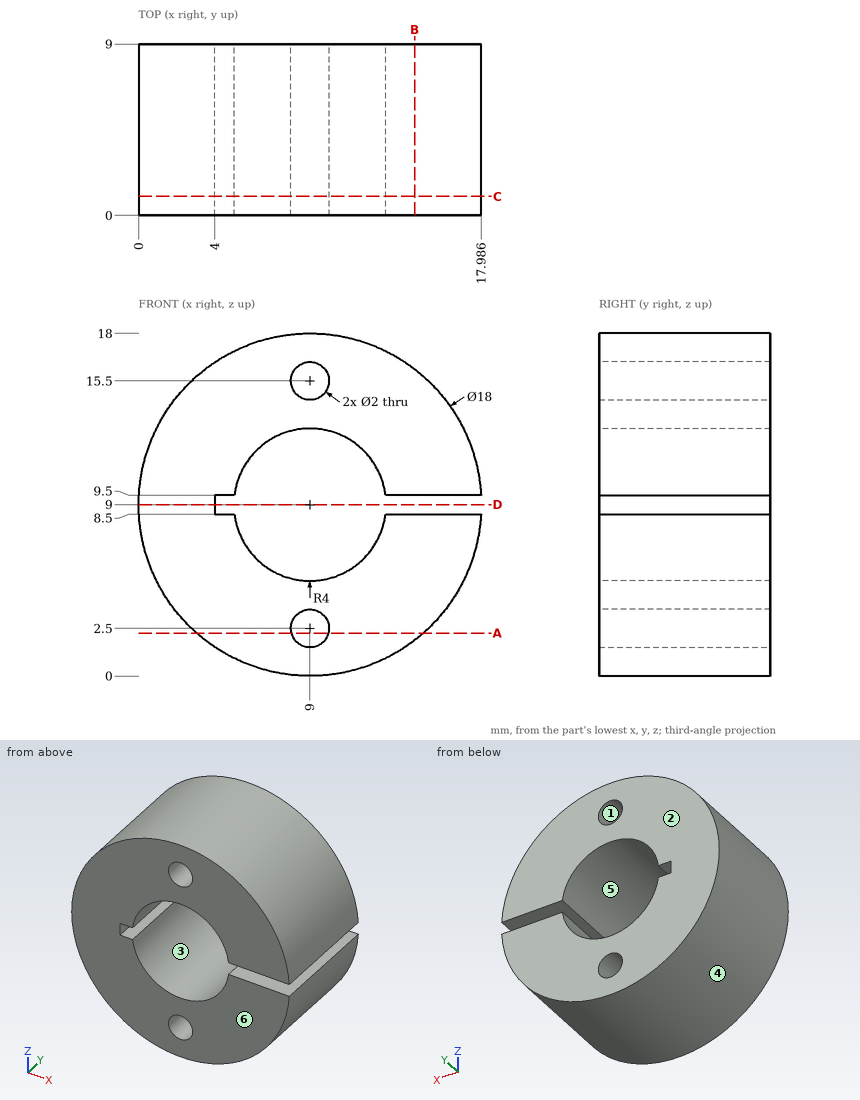
Verification items for this drawing (mm, ordinates from the low corner). A direction names the side the tool comes from. Coordinates: 2 decimals unless noted, no trailing zeros. Loops run counter-clockwise (first coordinate to the right, second up) from the corner with the lowest first, then second, coordinate; pieces in that order, holes last.
Item 1: Access from +Z, -Z, +X, -X, +Y, -Y to the whole of each face (thin tool, end or side, straight path). Record for the marked faces 5 and 6.
Item 2: Sectioned sample at B-B, the plane x = 14.5. Record the boundary of the cut face in (y, z), then the cut area to 3 significant figures.
Item 3: Release check for a two-part mould opening along X. For the marked faces 1, 2, 3 and 4 record: released by +X, released by -X, zero draft, split by the parting line, or undercut.
Item 4: Sectioned sample at D-D, the plane z = 9. Record the boundary of the cut face in (x, y).
Item 5: Sectioned sample at C-C, the plane y = 1. Record the boundary of the cut face in (x, z).
Item 6: Sectioned sample at A-A, the plane z = 2.25. Record the boundary of the cut face in (x, y), then the cut area to 3 significant figures.
Item 7: Go/stop test with flat-tipped pins: pin 1 Ø5 at (y, z) = (1.5, 14.5) entering from +X; pin 2 Ø2.5 at (x, z) = (9, 15.5) entering from -Y; pin 3 Ø1.5 at (x, y) = (15, 6.5) entering from +Z; pin 4 Ø0.8 at (y, z) = (5.5, 9) entering from +X. Record where each tip stops, or that it passes through.
Item 8: Thickness scan on line 1 (Z direction, x = 8.25, y = 5.75); line 2 (Z direction, x = 8.5, y = 3.5); line 3 (X direction, y = 2.5, z = 15.5) (1 decimal). Record the ranges inside material, lowest first.
Check result:
1. face 5: +Y, -Y
1. face 6: +Z, -Z, +X, -X, -Y
2. outline: (0, 1.88) - (9, 1.88) - (9, 8.5) - (0, 8.5) - close; (0, 9.5) - (9, 9.5) - (9, 16.12) - (0, 16.12) - close
2. area: 119 mm2
3. face 1: undercut
3. face 2: zero draft
3. face 3: undercut
3. face 4: split by the parting line
4. outline: (0, 0) - (4, 0) - (4, 9) - (0, 9) - close
5. outline: (4, 8.5) - (4, 9.5) - (5.03, 9.5) arc R4 cw to (12.97, 9.5) - (17.99, 9.5) arc R9 ccw (long way) to (17.99, 8.5) - (12.97, 8.5) arc R4 cw to (5.03, 8.5) - close; hole circle Ø2 at (9, 2.5); hole circle Ø2 at (9, 15.5)
6. outline: (3.05, 0) - (8.03, 0) - (8.03, 9) - (3.05, 9) - close; (9.97, 0) - (14.95, 0) - (14.95, 9) - (9.97, 9) - close
6. area: 89.7 mm2
7. pin 1: stops at x = 17.49
7. pin 2: stops at y = 0
7. pin 3: stops at z = 16.31
7. pin 4: stops at x = 4
8. line 1: z = 0.03 to 1.84, 3.16 to 5.07, 12.93 to 14.84, 16.16 to 17.97
8. line 2: z = 0.01 to 1.63, 3.37 to 5.03, 12.97 to 14.63, 16.37 to 17.99
8. line 3: x = 2.8 to 8, 10 to 15.2
